For this review, take the finished solid that the model builds, in its own axes (mm). Face numbers are marked on the shaded views. A direction names the side the tool comes from. Give positions to 0.01 mm unless a question says otherwise; leave off trailing zeros. Write each loop counter-clockwise with the first axis right and the second up, starting at its lowest first coordinate (ties: lowest second). Pieces come first, ordered by that corner, then holes.
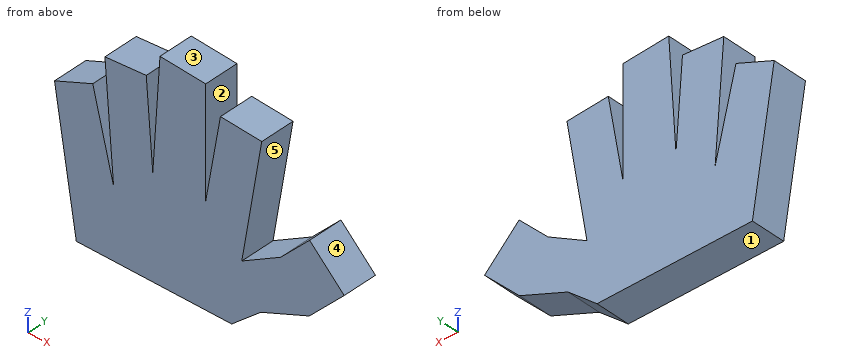
from build123d import *

# Parameters (mm, degrees)
F1_DEPTH = 5


with BuildPart() as f1:
    # F0 (on Front) → F1 (new body, symmetric)
    with BuildSketch(Plane.XZ):
        Polygon((-45, 0), (0, 0), (8.396735, 7.206781), (22.475777, 13.085932), (32.589957, 23.452093), (22.569422, 33.229049), (14.189174, 24.640019), (2.927364, 18.14605), (8.717845, 52.663731), (-3.256581, 53.446758), (-7.521497, 28.971553), (-7.521497, 60.037153), (-20.767864, 60.903354), (-22.855936, 28.971553), (-24.744828, 53.900092), (-36.710527, 52.993424), (-34.200146, 19.862823), (-40.235602, 44.123352), (-51.308924, 39.499335), align=None)
    extrude(amount=F1_DEPTH, both=True)


solid = f1.part
(1) We need section D-D (z = 47). Write out the cut boundary in (x, y), and give its area (3 significant figures).
(2) For L1, parallel to X at y = -2.5, z = 26; L2, parallel to X at y = -2.5, z = 51; L3, parallel to X at y = -1.5, z = 38.5, list the stretches that pass through material, from the lowest coordinate up.
(3) Tool access review of the marked faces 4 and 5: name each direction out of +Z, -Z, +X, -X, +Y, -Y from which nothing blocks a thin tool from reaching the whole face with its end or side.
(4) We need section A-A (y = 0.5). Write out the cut boundary in (x, z).
(5) We need section C-C (z = 35). Write out the cut boundary in (x, y), and give its area (3 significant figures).
(6) Clearance check with flat-ended pins moving along their axes: pin 1 Ø2 at (y, z) = (1.5, 45) entering from -X; pin 2 Ø3 at (y, z) = (1.5, 26.5) entering from -X; pin 3 Ø3 at (y, z) = (2, 42) entering from +X; pin 4 Ø2 at (x, y) = (-1, 0.5) entering from -Z. State where each tip first meets the part, or that it passes through.
(7) We need section B-B (x = 7). Write out the cut boundary in (y, z), and give its area (3 significant figures).
(8) The part is to be moulded in two halves that separate along X. For the marked faces 1, 2 and 3, say which applies: +X half, -X half, draft (parallel to the pull), parting line (faces both ways), or undercut.
The answers:
1. outline: (-36.26, -5) - (-24.22, -5) - (-24.22, 5) - (-36.26, 5) - close; (-21.68, -5) - (-7.52, -5) - (-7.52, 5) - (-21.68, 5) - close; (-4.38, -5) - (7.77, -5) - (7.77, 5) - (-4.38, 5) - close
1. area: 383 mm2
2. L1: x = -49.15 to -35.73, -34.67 to 4.24, 15.52 to 29.98
2. L2: x = -36.56 to -24.53, -21.42 to -7.52, -3.68 to 8.44
2. L3: x = -51.15 to -38.84, -35.61 to -23.58, -22.23 to -7.52, -5.86 to 6.34
3. face 4: +Z, +X, +Y, -Y
3. face 5: +Y, -Y
4. outline: (-51.31, 39.5) - (-45, 0) - (0, 0) - (8.4, 7.21) - (22.48, 13.09) - (32.59, 23.45) - (22.57, 33.23) - (14.19, 24.64) - (2.93, 18.15) - (8.72, 52.66) - (-3.26, 53.45) - (-7.52, 28.97) - (-7.52, 60.04) - (-20.77, 60.9) - (-22.86, 28.97) - (-24.74, 53.9) - (-36.71, 52.99) - (-34.2, 19.86) - (-40.24, 44.12) - close
5. outline: (-50.59, -5) - (-37.97, -5) - (-37.97, 5) - (-50.59, 5) - close; (-35.35, -5) - (-23.31, -5) - (-23.31, 5) - (-35.35, 5) - close; (-22.46, -5) - (-7.52, -5) - (-7.52, 5) - (-22.46, 5) - close; (-6.47, -5) - (5.75, -5) - (5.75, 5) - (-6.47, 5) - close
5. area: 518 mm2
6. pin 1: stops at x = -40.53
6. pin 2: stops at x = -49.47
6. pin 3: stops at x = 7.18
6. pin 4: stops at z = 0
7. outline: (-5, 6.01) - (5, 6.01) - (5, 20.49) - (-5, 20.49) - close; (-5, 42.42) - (5, 42.42) - (5, 52.78) - (-5, 52.78) - close
7. area: 248 mm2
8. face 1: draft
8. face 2: undercut
8. face 3: +X half
